Here's how the part is built. I have some questions about the finished solid (model axes, mm). Face numbers are marked on the shaded views. A direction names the side the tool comes from. Coordinates: 2 decimals unless noted, no trailing zeros. Loops run counter-clockwise (first coordinate to the right, second up) from the corner with the lowest first, then second, coordinate; pieces in that order, holes last.
from build123d import *

# Parameters (mm, degrees)
ESQUISSE1_R        = 3.75
ESQUISSE1_R_2      = 2.55
BOSS_EXTRU_1_DEPTH = 2
BOSS_EXTRU_2_START = 1
ESQUISSE2_R        = 3.75
BOSS_EXTRU_2_DEPTH = 1
ESQUISSE3_R        = 1.75
BOSS_EXTRU_3_DEPTH = 6
CONG_1_R           = 0.6
CHANFREIN1_SIZE    = 0.4
CHANFREIN2_SIZE    = 0.4


with BuildPart() as part:
    # Esquisse1 → Boss.-Extru.1 (new body)
    with BuildSketch(Plane.XY):
        Circle(ESQUISSE1_R)
        Circle(ESQUISSE1_R_2, mode=Mode.SUBTRACT)
    extrude(amount=BOSS_EXTRU_1_DEPTH)

    # Esquisse2 → Boss.-Extru.2 (add)
    with BuildSketch(Plane(origin=(0, 0, 0), x_dir=(-1, 0, 0), z_dir=(0, 0, -1)).offset(BOSS_EXTRU_2_START)):
        Circle(ESQUISSE2_R)
    extrude(amount=-BOSS_EXTRU_2_DEPTH)

    # Esquisse3 → Boss.-Extru.3 (add)
    with BuildSketch(Plane(origin=(0, 0, -1), x_dir=(-1, 0, 0), z_dir=(0, 0, -1))):
        Circle(ESQUISSE3_R)
    extrude(amount=BOSS_EXTRU_3_DEPTH)

    # Congé1
    cong_1_edges = [part.edges().sort_by_distance(p)[0] for p in [
        (1.75, 0, -1),
    ]]
    fillet(cong_1_edges, radius=CONG_1_R)

    # Chanfrein1
    chanfrein1_edges = [part.edges().sort_by_distance(p)[0] for p in [
        (1.75, 0, -7),
    ]]
    chamfer(chanfrein1_edges, length=CHANFREIN1_SIZE)

    # Chanfrein2
    chanfrein2_edges = [part.edges().sort_by_distance(p)[0] for p in [
        (-2.55, 0, 2),
    ]]
    chamfer(chanfrein2_edges, length=CHANFREIN2_SIZE)


solid = part.part
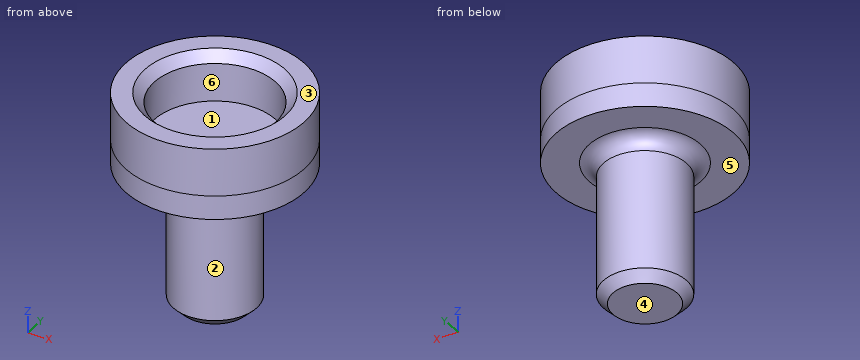
Q1. For the marked faces 4, 5 and 6, which set-ups out of +Z, -Z, +X, -X, +Y, -Y let a thin tool reach every point of the face, with its end or its side?
Q2. Suppose I cut it at A-A on x = 0. Write out the boundary of the cut face in (y, z).
Q3. Will these pins go through, and if not, where does the flat tip stop? P1, Ø1, axis at x = -2.5, y = -1, coming from the +Z side; P2, Ø4, axis at y = -3, z = -5.5, coming from the +X side.
Q4. Suppose I cut it at D-D on z = -5.5. Write out the boundary of the cut face in (x, y).
Q5. Please list where these lines run through material, in increasing order: probe 1 along Y at (x, z) = (0, 1.1); probe 2 along Z at (x, y) = (1.25, -0.25); probe 3 along Y at (x, z) = (-1.5, 0.75).
Q6. We'd pull the mould along Y, two halves only. Please class the marked faces 1, 2 and 3: pulls with the +Y half, pulls with the -Y half, needs draft (parallel to the pull), parting line crosses it, or undercut.
Q7. Suppose I cut it at C-C on z = 1.25. Write out the boundary of the cut face in (x, y).
Check values:
1. face 4: -Z, +X, -X, +Y, -Y
1. face 5: -Z
1. face 6: +Z
2. outline: (-3.75, -1) - (-2.35, -1) arc R0.6 cw to (-1.75, -1.6) - (-1.75, -6.6) - (-1.35, -7) - (1.35, -7) - (1.75, -6.6) - (1.75, -1.6) arc R0.6 cw to (2.35, -1) - (3.75, -1) - (3.75, 2) - (2.95, 2) - (2.55, 1.6) - (2.55, 0) - (-2.55, 0) - (-2.55, 1.6) - (-2.95, 2) - (-3.75, 2) - close
3. P1: stops at z = 2
3. P2: stops at x = 1.44
4. outline: circle Ø3.5 at (0, 0)
5. probe 1: y = -3.75 to -2.55, 2.55 to 3.75
5. probe 2: z = -7 to 0
5. probe 3: y = -3.44 to -2.06, 2.06 to 3.44
6. face 1: undercut
6. face 2: parting line crosses it
6. face 3: needs draft
7. outline: circle Ø7.5 at (0, 0); hole circle Ø5.1 at (0, 0)
